from build123d import *

# Parameters (mm, degrees)
F1_DEPTH = 8


with BuildPart() as f1:
    # F0 (on Front) → F1 (new body)
    with BuildSketch(Plane.XZ):
        with BuildLine():
            Line((72.5714285714, 14.7779482711), (4.6285714286, 26.6003068879))
            ThreePointArc((4.6285714286, 26.6003068879), (-27, 0), (4.6285714286, -26.6003068879))
            Line((4.6285714286, -26.6003068879), (72.5714285714, -14.7779482711))
            ThreePointArc((72.5714285714, -14.7779482711), (85, 0), (72.5714285714, 14.7779482711))
        make_face()
        Polygon((3.5863018887, 13.3842608598), (13.3842608598, 3.5863018887), (12.4233141649, 0), (9.7979589711, -9.7979589711), (-3.5863018887, -13.3842608598), (-13.3842608598, -3.5863018887), (-9.7979589711, 9.7979589711), align=None, mode=Mode.SUBTRACT)
        with BuildLine():
            ThreePointArc((78, 0), (70, -8), (62, 0))
            ThreePointArc((62, 0), (70, 8), (78, 0))
        make_face(mode=Mode.SUBTRACT)
    extrude(amount=F1_DEPTH)


solid = f1.part
Read the model definition and answer for the solid it produces. Units are mm, in the model's axes. A direction names the side the tool comes from. Give positions to 0.01 mm unless a question says otherwise; leave off trailing zeros. Loops run counter-clockwise (first coordinate to the right, second up) from the corner with the lowest first, then second, coordinate; pieces in that order, holes last. Notation, with made-up numbers: M -27,59 L -7,59 A14 ccw -7,81 Z; hole C 2.5,-8 d5. An arc over 180 degrees is marked long. Write each question's results on one line, items separated by ' | '.
1. Section C-C on x = 0 is taken. Give the vertices of the cut face in (y, z), plus the area to 3 significant figures.
Values:
outline: M -8,-27 L 0,-27 L 0,-12.42 L -8,-12.42 Z; M -8,12.42 L 0,12.42 L 0,27 L -8,27 Z | area: 233 mm^2
2. Given pin 1 (1.5 mm diameter, centred on y = -3.5, z = 9.5, fed in from +X); pin 2 (2 mm diameter, centred on y = -6, z = 4, fed in from -X); pin 3 (1.5 mm diameter, centred on y = -7, z = 2.5, fed in from +X), each flat-ended and moving along its own axis, determine where each tip first touches the part or whether it passes through.
Values:
pin 1: stops at x = 82.18 | pin 2: stops at x = -26.83 | pin 3: stops at x = 84.9
3. Section B-B on z = 0 is taken. Give the vertices of the cut face in (x, y), plus the area to 3 significant figures.
Values:
outline: M -27,-8 L -12.42,-8 L -12.42,0 L -27,0 Z; M 12.42,-8 L 62,-8 L 62,0 L 12.42,0 Z; M 78,-8 L 85,-8 L 85,0 L 78,0 Z | area: 569 mm^2
4. A tool of negligible diameter and unlimited length cuts with its end or side. For faces 1 (the face through (28, -8, 0)), 2 (the face through (8.42, -3.94, 8.55)), from which of +Z, -Z, +X, -X, +Y, -Y can it reach the whole face along a straight path? Write none if from no direction.
Values:
face 1: +Z, -Z, +X, -X, -Y | face 2: +Y, -Y
5. The mould has two halves that part along Z. Classify faces 3 (the face through (39.076, -3.944, 20.606)), 4 (the face through (-26.99, -3.94, 0.66)), 5 (the face through (3.2, -3.944, -11.566)), 6 (the face through (76.349, -3.944, -4.868)): pulls with the +Z half, pulls with the -Z half, needs draft (parallel to the pull), parting line crosses it, or undercut.
Values:
face 3: pulls with the +Z half | face 4: parting line crosses it | face 5: undercut | face 6: undercut
6. Section A-A on y = -6.5 is taken. Give the vertices of the cut face in (x, z).
Values:
outline: M 4.63,-26.6 L 72.57,-14.78 A15 ccw 72.57,14.78 L 4.63,26.6 A27 ccw long Z; hole M -13.38,-3.59 L -3.59,-13.38 L 9.8,-9.8 L 13.38,3.59 L 3.59,13.38 L -9.8,9.8 Z; hole C 70,0 d16
7. Straight lines are drawn through the part: line 1 (X direction, y = -6.25, z = -2); line 2 (X direction, y = -1, z = 0.5); line 3 (Z direction, x = 68, y = -3.5). For each, find the intervals that lie inside material, in ascending order. Write a range as [from, to].
Values:
line 1: x = [-26.93, -12.96], [11.89, 62.25], [77.75, 84.87] | line 2: x = [-27, -12.29], [12.56, 62.02], [77.98, 84.99] | line 3: z = [-15.57, -7.75], [7.75, 15.57]
8. Section D-D on z = 7 is taken. Give the vertices of the cut face in (x, y).
Values:
outline: M -26.08,-8 L -10.55,-8 L -10.55,0 L -26.08,0 Z; M 9.97,-8 L 66.13,-8 L 66.13,0 L 9.97,0 Z; M 73.87,-8 L 83.27,-8 L 83.27,0 L 73.87,0 Z
